Part print with two shaded views. Sizes in mm from the minimum x, y, z corner. A direction names the side the tool comes from. Round coordinates to 2 decimals unless told otherwise and drop trailing zeros. Loops run counter-clockwise (first coordinate to the right, second up) from the corner with the lowest first, then second, coordinate; pieces in that order, holes last. Notation, with made-up numbers: M 61,88.25 L 115,88.25 A26 ccw 115,118.25 Z; hole C -11,47.5 d8. An arc over 180 degrees is marked long. Use a Markdown table: item, result. Add a question column.
Item 1: Saw through at B-B on x = 10. Write the cut outline in (y, z).
Item 2: Tool access for the marked faces 1, 2 and 3: list every direction of +Z, -Z, +X, -X, +Y, -Y with a clear straight run to the whole face (end or side of a thin tool).
Item 3: Pin check, flat tips, straight feed: P1, Ø5, axis at y = 8.5, z = 37, coming from the +X side; P2, Ø6, axis at x = 28, y = 8.5, coming from the -Z side; P3, Ø6, axis at x = 44, y = 2.5, coming from the -Z side. Stop position of each tip, or through.
Item 4: Wall check: L1, parallel to Z at x = 18, y = 10; L2, parallel to Z at x = 66.5, y = 5 (1 decimal); L3, parallel to X at y = 1.25, z = 20.5 (1 decimal). Give the ranges that are in metal, low to high. Write a range as from..to.
Item 5: Saw through at C-C on z = 81. Write the cut outline in (x, y) (1 decimal), then the cut area to 3 significant figures.
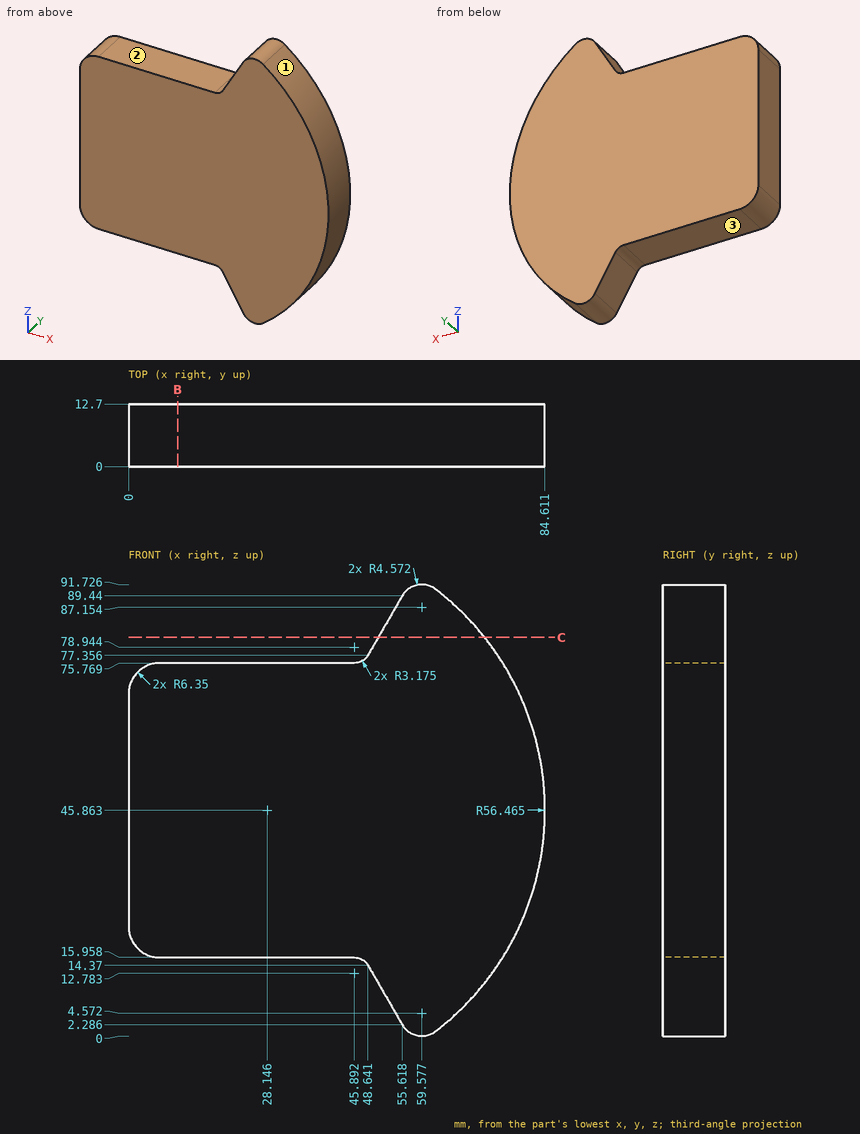
Entries:
| question | item | result |
|---|---|---|
| 1 | outline | M 0,15.96 L 12.7,15.96 L 12.7,75.77 L 0,75.77 Z |
| 2 | face 1 | +X, +Y, -Y |
| 2 | face 2 | +Z, -X, +Y, -Y |
| 2 | face 3 | -Z, -X, +Y, -Y |
| 3 | P1 | x = 84.25 |
| 3 | P2 | z = 15.96 |
| 3 | P3 | z = 15.76 |
| 4 | L1 | 15.96..75.77 |
| 4 | L2 | 4.4..87.3 |
| 4 | L3 | 0.3..78.6 |
| 5 | outline | M 50.7,0 L 72.3,0 L 72.3,12.7 L 50.7,12.7 Z |
| 5 | area | 274 mm2 |
